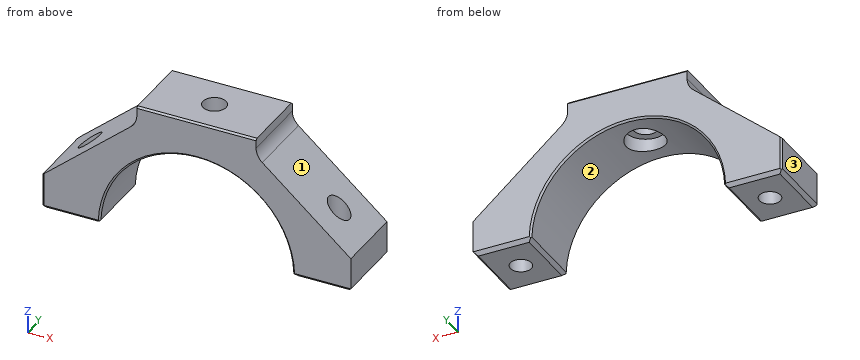
```python
from build123d import *

# Parameters (mm, degrees)
F1_DEPTH    = 20
F3_D        = 6
F4_T1_DEPTH = 21.6433659759
F4_T3_DEPTH = 21.6433659759
F4_T5_DEPTH = 25.0580427678
F4_T7_DEPTH = 25.1433659759
F5_SIZE     = 0.5
F7_D        = 6.6
F9_R        = 5.5
F10_DEPTH   = 3.5
F11_R       = 5


# Not quite as in the source:
# - a fillet or chamfer that OpenCascade refuses, or shapes differently, is made with other operations: its cross-section is extruded or revolved along the edge and cut away or added
# - a feature names something its author has since deleted; it is built from what else it names


with BuildPart() as f1:
    # F0 (on Front) → F1 (new body)
    with BuildSketch(Plane.XZ):
        with BuildLine():
            ThreePointArc((-27.5, 0), (0, 27.5), (27.5, 0))
            Line((27.5, 0), (44, 0))
            Line((44, 0), (44, 10))
            Line((44, 10), (17, 33))
            Line((17, 33), (17, 38))
            Line((17, 38), (-17, 38))
            Line((-17, 38), (-17, 33))
            Line((-17, 33), (-44, 10))
            Line((-44, 10), (-44, 0))
            Line((-44, 0), (-27.5, 0))
        make_face()
    extrude(amount=-F1_DEPTH)

    # F3 (through all)
    with Locations(Plane(origin=(0, 0, 0), x_dir=(1, 0, 0), z_dir=(0, 0, -1))):
        with Locations((-35.5, -10), (35.5, -10)):
            Hole(F3_D / 2)

    # F4: chamfer of 1 on 8 edges, made by hand

    # F4_s2 → F4_t1 (cut)
    with BuildSketch(Plane.YZ.offset(24.928317012)):
        Polygon((19, 0), (20, 1), (20, 0), align=None)
        Polygon((1, 0), (0, 1), (0, 0), align=None)
    extrude(amount=F4_T1_DEPTH, mode=Mode.SUBTRACT)

    # F4_s4 → F4_t3 (cut)
    with BuildSketch(Plane.YZ.offset(-46.571682988)):
        Polygon((19, 0), (20, 1), (20, 0), align=None)
        Polygon((1, 0), (0, 1), (0, 0), align=None)
    extrude(amount=F4_T3_DEPTH, mode=Mode.SUBTRACT)

    # F4_s6 → F4_t5 (cut)
    with BuildSketch(Plane.XZ.offset(-22.5290213839)):
        with BuildLine():
            Line((-27.4830665009, 0.9649122807), (-28.4824507373, 0))
            Line((-28.4824507373, 0), (-27.5, 0))
            ThreePointArc((-27.5, 0), (-27.4955143469, 0.4966797747), (-27.4830665009, 0.9649122807))
        make_face()
        with BuildLine():
            Line((27.4830665009, 0.9649122807), (28.4824507373, 0))
            Line((28.4824507373, 0), (27.5, 0))
            ThreePointArc((27.5, 0), (27.4955143469, 0.4966797747), (27.4830665009, 0.9649122807))
        make_face()
    extrude(amount=F4_T5_DEPTH, mode=Mode.SUBTRACT)

    # F4_s8 → F4_t7 (cut)
    with BuildSketch(Plane.XZ.offset(-22.571682988)):
        Polygon((-43, 0), (-44, 1), (-44, 0), align=None)
        Polygon((43, 0), (44, 1), (44, 0), align=None)
    extrude(amount=F4_T7_DEPTH, mode=Mode.SUBTRACT)

    # F5
    f5_edges = [f1.edges().sort_by_distance(p)[0] for p in [
        (0, 20, 38),
        (0, 0, 38),
        (0, 20, 27.5),
        (-44, 20, 5.5),
        (0, 0, 27.5),
        (-44, 0, 5.5),
    ]]
    chamfer(f5_edges, length=F5_SIZE)

    # F7 (through all)
    with Locations(Plane.XY.offset(38)):
        with Locations((0, 10)):
            Hole(F7_D / 2)

    # F9 (on offset) → F10 (cut, symmetric)
    with BuildSketch(Plane.XY.offset(27.5)):
        with Locations((0, 10)):
            Circle(F9_R)
    extrude(amount=F10_DEPTH, both=True, mode=Mode.SUBTRACT)

    # F11
    f11_edges = [f1.edges().sort_by_distance(p)[0] for p in [
        (-17, 10, 33),
        (17, 10, 33),
    ]]
    fillet(f11_edges, radius=F11_R)


solid = f1.part
```
The model under review builds one solid part; all positions refer to its coordinate system, in mm. Face numbers are marked on the shaded views. Round coordinates to 2 decimals unless told otherwise and drop trailing zeros. Loops run counter-clockwise (first coordinate to the right, second up) from the corner with the lowest first, then second, coordinate; pieces in that order, holes last. Notation, with made-up numbers: (84.25, 23) - (88.25, 23) arc R24 cw to (88.25, 37) - close; hole circle Ø7 at (-38.75, -23). An arc over 180 degrees is marked (long way). Write each question's results on one line, items separated by ' | '. Start each with the question number.
Q1. Wall thickness on line 1 along X through (y, z) = (10, 6.5); line 2 along X through (y, z) = (10, 14.5); line 3 along X through (y, z) = (18.25, 4.5): over which ranges is each line inside the solid? List them lowest first. Write a range as [from, to].
Q2. Take a section at C-C on z = 3. Give the number of separate pieces and of enclosed holes in the cut face, plus the area to 3 significant figures.
Q3. Draft analysis for pull direction X (two halves, no side actions). For the marked faces 1, 2 and 3, state which applies: pulls with the +X half, pulls with the -X half, needs draft (parallel to the pull), parting line crosses it, or undercut.
Q4. Take a section at B-B on y = 3. Give the boundary of the cut face in (x, z), plus the area to 3 significant figures.
Q5. Take a section at A-A on x = 35.5. Give the boundary of the cut face in (y, z).
Q6. Insertion check: P1, Ø5.5, axis at x = 2, y = 11.5, coming from the -Z side; P2, Ø12, axis at y = 3.5, z = 19.5, coming from the +X side; P3, Ø7, axis at x = 35.5, y = 10, coming from the +Z side; P4, Ø3.5, axis at x = -35.5, y = 10, coming from the -Z side. Each pin has a flat end and moves straight along its axis. Give the tip position at first contact, or say it passes through.
Data:
1) line 1: x = [-44, -38.5], [-32.5, -26.72], [26.72, 32.5], [38.5, 44] | line 2: x = [-38.72, -38.5], [-32.5, -23.37], [23.37, 32.5], [38.5, 38.72] | line 3: x = [-44, -27.13], [27.13, 44]
2) separate pieces: 2 | enclosed holes: 2 | area: 609 mm²
3) face 1: pulls with the +X half | face 2: undercut | face 3: pulls with the -X half
4) outline: (-44, 1) - (-43, 0) - (-28.48, 0) - (-27.48, 0.96) arc R27.5 cw to (27.48, 0.96) - (28.48, 0) - (43, 0) - (44, 1) - (44, 10) - (18.76, 31.5) arc R5 cw to (17, 35.31) - (17, 38) - (-17, 38) - (-17, 35.31) arc R5 cw to (-18.76, 31.5) - (-44, 10) - close | area: 1,260 mm²
5) outline: (0, 1) - (1, 0) - (7, 0) - (7, 17.24) - (0, 17.24) - close; (13, 0) - (19, 0) - (20, 1) - (20, 17.24) - (13, 17.24) - close
6) P1: stops at z = 31 | P2: stops at x = 39.89 | P3: stops at z = 20.22 | P4: passes through
